from build123d import *

# Parameters (mm, degrees)
Y_KSEKLIK_EKSTR_ZYON1_DEPTH = 2
RADYUS1_R                   = 10
RADYUS2_R                   = 3


with BuildPart() as part:
    # Çizim1 → Yükseklik-Ekstrüzyon1 (new body)
    with BuildSketch(Plane.XY):
        Polygon((78.397764574, 53), (78.397764574, 58), (-79.202235426, 58), (-79.202235426, 53), (-79.202235426, 4.7), (-99.202235426, 4.7), (-99.202235426, -129.7), (-79.202235426, -129.7), (-79.202235426, -178), (-79.202235426, -183), (78.397764574, -183), (78.397764574, -178), (78.397764574, -129.7), (98.397764574, -129.7), (98.397764574, 4.7), (78.397764574, 4.7), align=None)
    extrude(amount=Y_KSEKLIK_EKSTR_ZYON1_DEPTH)

    # Radyus1
    radyus1_edges = [part.edges().sort_by_distance(p)[0] for p in [
        (-79.202235426, 58, 1),
        (78.397764574, 58, 1),
        (98.397764574, 4.7, 1),
        (98.397764574, -129.7, 1),
        (78.397764574, -183, 1),
        (-79.202235426, -183, 1),
        (-99.202235426, -129.7, 1),
        (-99.202235426, 4.7, 1),
    ]]
    fillet(radyus1_edges, radius=RADYUS1_R)

    # Radyus2
    radyus2_edges = [part.edges().sort_by_distance(p)[0] for p in [
        (78.397764574, 4.7, 1),
        (78.397764574, -129.7, 1),
        (-79.202235426, -129.7, 1),
        (-79.202235426, 4.7, 1),
    ]]
    fillet(radyus2_edges, radius=RADYUS2_R)


solid = part.part
Can you work these out from the model? Positions are in its coordinate system, mm. Give positions to 0.01 mm unless a question says otherwise; leave off trailing zeros. Order: outer loops, then holes, each group sorted by start corner. A loop starts at its lowest first (then second) coordinate and runs counter-clockwise, first axis right, second up. Notation, with made-up numbers: M -10,22 L -5,22 A18 ccw -5,35 Z; hole C -8,24 d11. An arc over 180 degrees is marked long. One line per question, with ' | ' between items.
Item 1: Please list where these lines run through material, in increasing order: L1, parallel to X at y = -120.5, z = 0.6; L2, parallel to Y at x = -82, z = 0.4; L3, parallel to X at y = -124.5, z = 1.4.
Answer block:
L1: x = -99.17 to 98.37 | L2: y = -129.71 to 4.71 | L3: x = -97.97 to 97.17
Item 2: Suppose I cut it at A-A, the plane z = 0.8. Write out the boundary of the cut face in (x, y).
Answer block:
outline: M -99.2,-119.7 A10 ccw -89.2,-129.7 L -82.2,-129.7 A3 cw -79.2,-132.7 L -79.2,-173 A10 ccw -69.2,-183 L 68.4,-183 A10 ccw 78.4,-173 L 78.4,-132.7 A3 cw 81.4,-129.7 L 88.4,-129.7 A10 ccw 98.4,-119.7 L 98.4,-5.3 A10 ccw 88.4,4.7 L 81.4,4.7 A3 cw 78.4,7.7 L 78.4,48 A10 ccw 68.4,58 L -69.2,58 A10 ccw -79.2,48 L -79.2,7.7 A3 cw -82.2,4.7 L -89.2,4.7 A10 ccw -99.2,-5.3 Z
Item 3: Suppose I cut it at B-B, the plane y = -139.5. Write out the boundary of the cut face in (x, z), then the cut area to 3 significant figures.
Answer block:
outline: M -79.2,0 L 78.4,0 L 78.4,2 L -79.2,2 Z | area: 315 mm2
Item 4: I'm going to push flat-ended pins straight in: pin 1 Ø4 at (x, y) = (29.5, -128) entering from -Z; pin 2 Ø1 at (y, z) = (35.5, 0.5) entering from -X; pin 3 Ø0.6 at (x, z) = (83.5, 1) entering from -Y; pin 4 Ø1 at (y, z) = (-146.5, 0.5) entering from +X. Where does each tip first touch, or does it pass through?
Answer block:
pin 1: stops at z = 0 | pin 2: stops at x = -79.2 | pin 3: stops at y = -129.7 | pin 4: stops at x = 78.4
